Input: part model. Units: mm. Frame: model coordinates. Coordinates: 2 decimals unless noted, no trailing zeros. Loops run counter-clockwise (first coordinate to the right, second up) from the corner with the lowest first, then second, coordinate; pieces in that order, holes last. Notation, with made-up numbers: (81.5, 3.5) -> (100.5, 3.5) arc R26 ccw to (100.5, 32.5) -> close; hole circle Ø2 at (59, 21.5). An arc over 180 degrees is marked (long way). Answer as a JSON object with one key per item and string values.
Autodesk Inventor part; units mm, degrees
ref_plane "YZ Plane" through (0, 0, 0) normal (1, 0, 0) x (0, 1, 0)
ref_plane "XZ Plane" through (0, 0, 0) normal (0, 1, 0) x (-1, 0, 0)
ref_plane "XY Plane" through (0, 0, 0) normal (0, 0, 1) x (1, 0, 0)
sketch "Sketch1" plane through (0, 0, 0) normal (0, 1, 0) x (-1, 0, 0)
  circle A0 centre (0, 0) radius 45.72
  dimension "d0" = 91.44
extrude "Extrusion1" add sketch "Sketch1" along normal blind 5.588
sketch "Sketch2" plane through (0, 5.588, 0) normal (0, 1, 0) x (1, 0, 0)
  circle A0 centre (0, 0) radius 38.1
  line L0 (0, 0) -> (-41.91, 0)
  line L1 (0, 0) -> (0, 41.91)
  line L2 (0, 0) -> (41.91, 0)
  line L3 (0, 0) -> (0, -41.91)
  circle A1 centre (-41.91, 0) radius 1.27
  circle A2 centre (0, 41.91) radius 1.27
  circle A3 centre (41.91, 0) radius 1.27
  circle A4 centre (0, -41.91) radius 1.27
  dimension "d3" = 76.2
  dimension "d4" = 41.91
  dimension "d5" = 41.91
  dimension "d6" = 41.91
  dimension "d7" = 41.91
  dimension "d8" = 2.54
  dimension "d9" = 2.54
  dimension "d10" = 2.54
  dimension "d11" = 2.54
extrude "Extrusion2" cut sketch "Sketch2" against normal blind 5.588
properties part number "open3" material "Plastic, Transparent"
1. Section query C-C (y = 4). Return loops of the section in (x, z).
Reply:
{"outline": "circle Ø91.44 at (0, 0); hole circle Ø2.54 at (-41.91, 0); hole circle Ø76.2 at (0, 0); hole circle Ø2.54 at (0, -41.91); hole circle Ø2.54 at (0, 41.91); hole circle Ø2.54 at (41.91, 0)"}
2. Pin query (flat end, axial travel): P1, Ø3, axis at y = 5, z = 34.5, coming from the +X side; P2, Ø2, axis at x = -21.5, y = 4, coming from the -Z side; P3, Ø3, axis at x = 12.5, y = 1.5, coming from the +Z side. Return the tip coordinate at first contact, or that it passes through.
Reply:
{"P1": "stops at x = 31.64", "P2": "stops at z = -40.87", "P3": "stops at z = 44.38"}
3. Section query A-A (z = 0). Return loops of the section in (x, y).
Reply:
{"outline": "(-45.72, 0) -> (-43.18, 0) -> (-43.18, 5.59) -> (-45.72, 5.59) -> close; (-40.64, 0) -> (-38.1, 0) -> (-38.1, 5.59) -> (-40.64, 5.59) -> close; (38.1, 0) -> (40.64, 0) -> (40.64, 5.59) -> (38.1, 5.59) -> close; (43.18, 0) -> (45.72, 0) -> (45.72, 5.59) -> (43.18, 5.59) -> close"}
4. Section query B-B (x = 0). Return loops of the section in (y, z).
Reply:
{"outline": "(0, -45.72) -> (5.59, -45.72) -> (5.59, -43.18) -> (0, -43.18) -> close; (0, -40.64) -> (5.59, -40.64) -> (5.59, -38.1) -> (0, -38.1) -> close; (0, 38.1) -> (5.59, 38.1) -> (5.59, 40.64) -> (0, 40.64) -> close; (0, 43.18) -> (5.59, 43.18) -> (5.59, 45.72) -> (0, 45.72) -> close"}
5. Mould query, pull axis Z, two halves, no side actions, for faces 1 (the face through (-0.17, 2.83, -43.17)), 2 (the face through (-43.61, 2.75, -13.73)), 3 (the face through (-10, 0, -37)). Classes: pulls with the +Z half, pulls with the -Z half, needs draft (parallel to the pull), parting line crosses it, or undercut.
Reply:
{"face 1": "undercut", "face 2": "parting line crosses it", "face 3": "needs draft"}
6. Section query D-D (z = -41.91). Return loops of the section in (x, y).
Reply:
{"outline": "(-18.27, 0) -> (-1.27, 0) -> (-1.27, 5.59) -> (-18.27, 5.59) -> close; (1.27, 0) -> (18.27, 0) -> (18.27, 5.59) -> (1.27, 5.59) -> close"}
7. Line query: line 1 along Z through (x, y) = (0, 4.25); line 2 along X through (y, z) = (4.35, -41.91); line 3 along Z through (x, y) = (-34.5, 4.1). Output: solid intervals per line, ascending.
Reply:
{"line 1": "z = -45.72 to -43.18, -40.64 to -38.1, 38.1 to 40.64, 43.18 to 45.72", "line 2": "x = -18.27 to -1.27, 1.27 to 18.27", "line 3": "z = -30 to -16.17, 16.17 to 30"}
